```python
from build123d import *

# Parameters (mm, degrees)
SKETCH1_R           = 2.5
BOSS_EXTRUDE1_DEPTH = 250


with BuildPart() as part:
    # Sketch1 → Boss-Extrude1 (new body)
    with BuildSketch(Plane.XY):
        with BuildLine():
            Line((-3.6, -10), (-8.5, -10))
            ThreePointArc((-8.5, -10), (-9.560660172, -9.560660172), (-10, -8.5))
            Line((-10, -8.5), (-10, -3.5))
            Line((-10, -3.5), (-9.4, -3.5))
            Line((-9.4, -3.5), (-9.4, -3))
            Line((-9.4, -3), (-8.2, -3))
            Line((-8.2, -3), (-8.2, -5.4))
            Line((-8.2, -5.4), (-7.081980515, -5.4))
            ThreePointArc((-7.081980515, -5.4), (-6.507955367, -5.285819299), (-6.021320344, -4.960660172))
            Line((-6.021320344, -4.960660172), (-4.339339828, -3.278679656))
            ThreePointArc((-4.339339828, -3.278679656), (-4.014180701, -2.792044633), (-3.9, -2.218019485))
            Line((-3.9, -2.218019485), (-3.9, 2.218019485))
            ThreePointArc((-3.9, 2.218019485), (-4.014180701, 2.792044633), (-4.339339828, 3.278679656))
            Line((-4.339339828, 3.278679656), (-6.021320344, 4.960660172))
            ThreePointArc((-6.021320344, 4.960660172), (-6.507955367, 5.285819299), (-7.081980515, 5.4))
            Line((-7.081980515, 5.4), (-8.2, 5.4))
            Line((-8.2, 5.4), (-8.2, 3))
            Line((-8.2, 3), (-9.4, 3))
            Line((-9.4, 3), (-9.4, 3.5))
            Line((-9.4, 3.5), (-10, 3.5))
            Line((-10, 3.5), (-10, 8.5))
            ThreePointArc((-10, 8.5), (-9.560660172, 9.560660172), (-8.5, 10))
            Line((-8.5, 10), (-3.6, 10))
            Line((-3.6, 10), (-3.6, 9.4))
            Line((-3.6, 9.4), (-3.1, 9.4))
            Line((-3.1, 9.4), (-3.1, 8.2))
            Line((-3.1, 8.2), (-5.5, 8.2))
            Line((-5.5, 8.2), (-5.5, 7.181980515))
            ThreePointArc((-5.5, 7.181980515), (-5.385819299, 6.607955367), (-5.060660172, 6.121320344))
            Line((-5.060660172, 6.121320344), (-3.278679656, 4.339339828))
            ThreePointArc((-3.278679656, 4.339339828), (-2.792044633, 4.014180701), (-2.218019485, 3.9))
            Line((-2.218019485, 3.9), (2.218019485, 3.9))
            ThreePointArc((2.218019485, 3.9), (2.792044633, 4.014180701), (3.278679656, 4.339339828))
            Line((3.278679656, 4.339339828), (5.060660172, 6.121320344))
            ThreePointArc((5.060660172, 6.121320344), (5.385819299, 6.607955367), (5.5, 7.181980515))
            Line((5.5, 7.181980515), (5.5, 8.2))
            Line((5.5, 8.2), (3.1, 8.2))
            Line((3.1, 8.2), (3.1, 9.4))
            Line((3.1, 9.4), (3.6, 9.4))
            Line((3.6, 9.4), (3.6, 10))
            Line((3.6, 10), (8.5, 10))
            ThreePointArc((8.5, 10), (9.560660172, 9.560660172), (10, 8.5))
            Line((10, 8.5), (10, 3.5))
            Line((10, 3.5), (9.4, 3.5))
            Line((9.4, 3.5), (9.4, 3))
            Line((9.4, 3), (8.2, 3))
            Line((8.2, 3), (8.2, 5.4))
            Line((8.2, 5.4), (7.081980515, 5.4))
            ThreePointArc((7.081980515, 5.4), (6.507955367, 5.285819299), (6.021320344, 4.960660172))
            Line((6.021320344, 4.960660172), (4.339339828, 3.278679656))
            ThreePointArc((4.339339828, 3.278679656), (4.014180701, 2.792044633), (3.9, 2.218019485))
            Line((3.9, 2.218019485), (3.9, -2.218019485))
            ThreePointArc((3.9, -2.218019485), (4.014180701, -2.792044633), (4.339339828, -3.278679656))
            Line((4.339339828, -3.278679656), (6.021320344, -4.960660172))
            ThreePointArc((6.021320344, -4.960660172), (6.507955367, -5.285819299), (7.081980515, -5.4))
            Line((7.081980515, -5.4), (8.2, -5.4))
            Line((8.2, -5.4), (8.2, -3))
            Line((8.2, -3), (9.4, -3))
            Line((9.4, -3), (9.4, -3.5))
            Line((9.4, -3.5), (10, -3.5))
            Line((10, -3.5), (10, -8.5))
            ThreePointArc((10, -8.5), (9.560660172, -9.560660172), (8.5, -10))
            Line((8.5, -10), (3.6, -10))
            Line((3.6, -10), (3.6, -9.4))
            Line((3.6, -9.4), (3.1, -9.4))
            Line((3.1, -9.4), (3.1, -8.2))
            Line((3.1, -8.2), (5.5, -8.2))
            Line((5.5, -8.2), (5.5, -7.181980515))
            ThreePointArc((5.5, -7.181980515), (5.385819299, -6.607955367), (5.060660172, -6.121320344))
            Line((5.060660172, -6.121320344), (3.278679656, -4.339339828))
            ThreePointArc((3.278679656, -4.339339828), (2.792044633, -4.014180701), (2.218019485, -3.9))
            Line((2.218019485, -3.9), (-2.218019485, -3.9))
            ThreePointArc((-2.218019485, -3.9), (-2.792044633, -4.014180701), (-3.278679656, -4.339339828))
            Line((-3.278679656, -4.339339828), (-5.060660172, -6.121320344))
            ThreePointArc((-5.060660172, -6.121320344), (-5.385819299, -6.607955367), (-5.5, -7.181980515))
            Line((-5.5, -7.181980515), (-5.5, -8.2))
            Line((-5.5, -8.2), (-3.1, -8.2))
            Line((-3.1, -8.2), (-3.1, -9.4))
            Line((-3.1, -9.4), (-3.6, -9.4))
            Line((-3.6, -9.4), (-3.6, -10))
        make_face()
        Circle(SKETCH1_R, mode=Mode.SUBTRACT)
    extrude(amount=BOSS_EXTRUDE1_DEPTH)


solid = part.part
```
Source: CAD feature listing. Evaluate the final solid. Frame: model axes, mm. A direction names the side the tool comes from. Round coordinates to 2 decimals unless told otherwise and drop trailing zeros. Order: outer loops, then holes, each group sorted by start corner. A loop starts at its lowest first (then second) coordinate and runs counter-clockwise, first axis right, second up. Notation, with made-up numbers: (38.25, 15) -> (63.25, 15) arc R16 cw to (63.25, 37) -> close; hole circle Ø3 at (55.25, 47). An arc over 180 degrees is marked (long way). One line per item, written item: value. Start each with the question number.
Q1. Pin query (flat end, axial travel): pin 1 (4 mm diameter, centred on y = -2, z = 148.5, fed in from -X); pin 2 (1 mm diameter, centred on y = 0, z = 133, fed in from +X); pin 3 (0.7 mm diameter, centred on x = -9.5, z = 145, fed in from +Y); pin 4 (0.6 mm diameter, centred on y = 9, z = 148.5, fed in from +X). Return the tip coordinate at first contact, or that it passes through.
Q2. Section query A-A (x = 0). Return the cut outline in (y, z).
Q3. Access query for faces 5 (the flat face through (0, 3.9, 123)), 6 (the flat face through (0, -3.9, 123)), 7 (the flat face through (2, -2, 0)). Directions: +Z, -Z, +X, -X, +Y, -Y. A direction counts if a zero-diameter tool reaches every point of the face in a straight line with its end or side. Return the directions, or none.
Q4. Draft query along Y for faces 1 (the flat face through (10, 6, 123)), 2 (the flat face through (-6, 10, 123)), 3 (the flat face through (-3.9, 0, 123)), 4 (the flat face through (3.9, 0, 123)). Return one class per face: pulls with the +Y half, pulls with the -Y half, needs draft (parallel to the pull), parting line crosses it, or undercut.
Q5. Material intervals for probe 1 along X at (y, z) = (7.75, 169.5); probe 2 along Y at (x, z) = (-0.25, 221); probe 3 along Y at (x, z) = (-4.75, 221.5), sorted ascending.
Findings below:
1. pin 1: x = -10
1. pin 2: x = 3.9
1. pin 3: y = 9.85
1. pin 4: x = 9.99
2. outline: (-3.9, 0) -> (-2.5, 0) -> (-2.5, 250) -> (-3.9, 250) -> close; (2.5, 0) -> (3.9, 0) -> (3.9, 250) -> (2.5, 250) -> close
3. face 5: +Z, -Z, +Y
3. face 6: +Z, -Z, -Y
3. face 7: -Z, +X, -X, +Y, -Y
4. face 1: needs draft
4. face 2: pulls with the +Y half
4. face 3: undercut
4. face 4: undercut
5. probe 1: -10 to -5.5, 5.5 to 10
5. probe 2: -3.9 to -2.49, 2.49 to 3.9
5. probe 3: -10 to -8.2, -5.81 to -3.69, 3.69 to 5.81, 8.2 to 10
